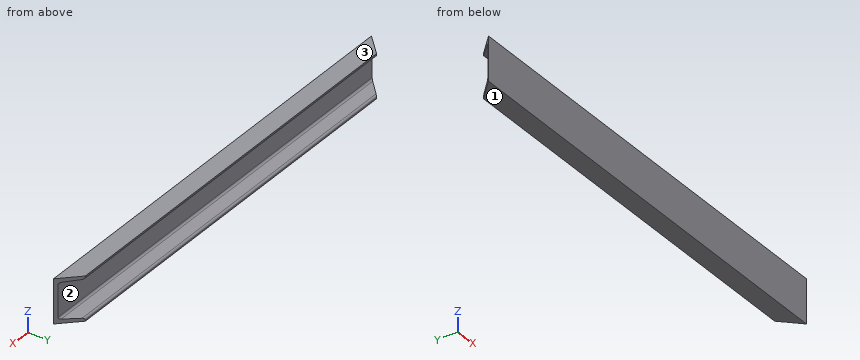
```python
from build123d import *

# Parameters (mm, degrees)
F1_DEPTH = 1000
F3_DEPTH = 100.001
F5_DEPTH = 100.001


with BuildPart() as f1:
    # F0 (on Right) → F1 (new body)
    with BuildSketch(Plane.YZ):
        with BuildLine():
            Line((0, 100), (0, 0))
            Line((0, 0), (42, 0))
            Line((42, 0), (42, 2.664711))
            ThreePointArc((42, 2.664711), (40.806503, 5.717093), (37.859095, 7.150361))
            Line((37.859095, 7.150361), (10.140905, 9.369315))
            ThreePointArc((10.140905, 9.369315), (7.193497, 10.802582), (6, 13.854964))
            Line((6, 13.854964), (6, 86.145036))
            ThreePointArc((6, 86.145036), (7.193497, 89.197418), (10.140905, 90.630685))
            Line((10.140905, 90.630685), (37.859095, 92.849639))
            ThreePointArc((37.859095, 92.849639), (40.806503, 94.282907), (42, 97.335289))
            Line((42, 97.335289), (42, 100))
            Line((42, 100), (0, 100))
        make_face()
    extrude(amount=F1_DEPTH)

    # F2 (on face) → F3 (cut, through all)
    with BuildSketch(Plane.XY.offset(100)):
        Polygon((958, 42), (1000, 0), (1000, 42), align=None)
    extrude(amount=-F3_DEPTH, mode=Mode.SUBTRACT)

    # F4 (on face) → F5 (cut, through all)
    with BuildSketch(Plane.XY.offset(100)):
        Polygon((0, 42), (0, 0), (42, 42), align=None)
    extrude(amount=-F5_DEPTH, mode=Mode.SUBTRACT)


solid = f1.part
```
Part model, mm, in its own coordinate system. Face numbers are marked on the shaded views. Round coordinates to 2 decimals unless told otherwise and drop trailing zeros. Loops run counter-clockwise (first coordinate to the right, second up) from the corner with the lowest first, then second, coordinate; pieces in that order, holes last.
1. Slice it at C-C (z = 51.5). Give the cut face in (x, y), and give its area (3 significant figures).
Solutions:
outline: (0, 0) - (1000, 0) - (994, 6) - (6, 6) - close
area: 5,960 mm2
2. Flat gauge pin, fed straight in: pin 1 (8 mm diameter, centred on x = 706.5, z = 58, fed in from +Y). Where does the tip first touch, or does it go through?
Solutions:
pin 1: stops at y = 6
3. Drill centre lines: line 1 along Y through (x, z) = (492, 36.5); line 2 along Z through (x, y) = (848, 11.5); line 3 along Z through (x, y) = (440, 16.5). Where is each one in solid material? Low to high.
Solutions:
line 1: y = 0 to 6
line 2: z = 0 to 9.26, 90.74 to 100
line 3: z = 0 to 8.86, 91.14 to 100
4. Slice it at A-A (x = 289). Give the cut face in (y, z).
Solutions:
outline: (0, 0) - (42, 0) - (42, 2.66) arc R4.5 ccw to (37.86, 7.15) - (10.14, 9.37) arc R4.5 cw to (6, 13.85) - (6, 86.15) arc R4.5 cw to (10.14, 90.63) - (37.86, 92.85) arc R4.5 ccw to (42, 97.34) - (42, 100) - (0, 100) - close
5. Slice it at B-B (y = 27). Give the cut face in (x, z).
Solutions:
outline: (27, 0) - (973, 0) - (973, 8.02) - (27, 8.02) - close; (27, 91.98) - (973, 91.98) - (973, 100) - (27, 100) - close
6. Two-plate mould, pull along Z, no slides. Class the marked faces 1, 2 and 3: pulls with the +Z half, pulls with the -Z half, needs draft (parallel to the pull), parting line crosses it, or undercut.
Solutions:
face 1: pulls with the -Z half
face 2: undercut
face 3: pulls with the +Z half
